CAD build for the part. Positions are in the model's coordinates, mm. A direction names the side the tool comes from. Give positions to 0.01 mm unless a question says otherwise; leave off trailing zeros. Loops run counter-clockwise (first coordinate to the right, second up) from the corner with the lowest first, then second, coordinate; pieces in that order, holes last.
```python
from build123d import *

# Parameters (mm, degrees)
ESQUISSE1_R        = 5
BOSS_EXTRU_1_DEPTH = 25
ESQUISSE2_R        = 2.755
BOSS_EXTRU_2_DEPTH = 5
BOSS_EXTRU_3_START = 5
ESQUISSE3_R        = 2.755
BOSS_EXTRU_3_DEPTH = 5
CONG_2_R           = 2
CONG_3_R           = 2


with BuildPart() as part:
    # Esquisse1 → Boss.-Extru.1 (new body)
    with BuildSketch(Plane.XY):
        Circle(ESQUISSE1_R)
    extrude(amount=BOSS_EXTRU_1_DEPTH)

    # Esquisse2 → Boss.-Extru.2 (add)
    with BuildSketch(Plane.XY.offset(25)):
        Circle(ESQUISSE2_R)
    extrude(amount=BOSS_EXTRU_2_DEPTH)

    # Esquisse3 → Boss.-Extru.3 (add)
    with BuildSketch(Plane(origin=(0, 0, 0), x_dir=(-1, 0, 0), z_dir=(0, 0, -1)).offset(BOSS_EXTRU_3_START)):
        with Locations(Location((0, 0, 0), (0, 0, 180))):
            Circle(ESQUISSE3_R)
    extrude(amount=-BOSS_EXTRU_3_DEPTH)

    # Congé2
    cong_2_edges = [part.edges().sort_by_distance(p)[0] for p in [
        (-5, 0, 0),
    ]]
    fillet(cong_2_edges, radius=CONG_2_R)

    # Congé3
    cong_3_edges = [part.edges().sort_by_distance(p)[0] for p in [
        (-5, 0, 25),
    ]]
    fillet(cong_3_edges, radius=CONG_3_R)


solid = part.part
```
1. Drop flat-ended pins along their axis: pin 1 (5 mm diameter, centred on x = 3.5, z = 0, fed in from +Y); pin 2 (4 mm diameter, centred on x = 3, z = 14, fed in from -Y); pin 3 (3 mm diameter, centred on x = 3.5, y = 4, fed in from -Z). Give the stop position or say it passes through.
Responses:
pin 1: stops at y = 4.7
pin 2: stops at y = -4.9
pin 3: stops at z = 0.17
2. Saw through at A-A, the plane x = 0. List the corners of the cut face in (y, z) (3 decimals), and give its area (3 significant figures).
Responses:
outline: (-5, 2) arc R2 ccw to (-3, 0) - (-2.755, 0) - (-2.755, -5) - (2.755, -5) - (2.755, 0) - (3, 0) arc R2 ccw to (5, 2) - (5, 23) arc R2 ccw to (3, 25) - (2.755, 25) - (2.755, 30) - (-2.755, 30) - (-2.755, 25) - (-3, 25) arc R2 ccw to (-5, 23) - close
area: 302 mm2
3. Saw through at B-B, the plane z = 23.5. List the corners of the cut face in (x, y).
Responses:
outline: circle Ø9.87 at (0, 0)
4. Tool access for faces 1 (the face through (-1.08, -4.88, 12.35)), 2 (the face through (2.628, -0.828, -2.535)), 3 (the face through (2.628, 0.828, 27.465)): list every direction of +Z, -Z, +X, -X, +Y, -Y with a clear straight run to the whole face (end or side of a thin tool).
Responses:
face 1: +Z, -Z
face 2: -Z
face 3: +Z
5. Probe line 1 along X through (y, z) = (0.25, 11); line 2 along Z through (x, y) = (2.75, 0.5); line 3 along Y through (x, z) = (-4, 2). List the from-to ranges inside material, lowest first.
Responses:
line 1: x = -4.99 to 4.99
line 2: z = 0 to 25
line 3: y = -3 to 3
